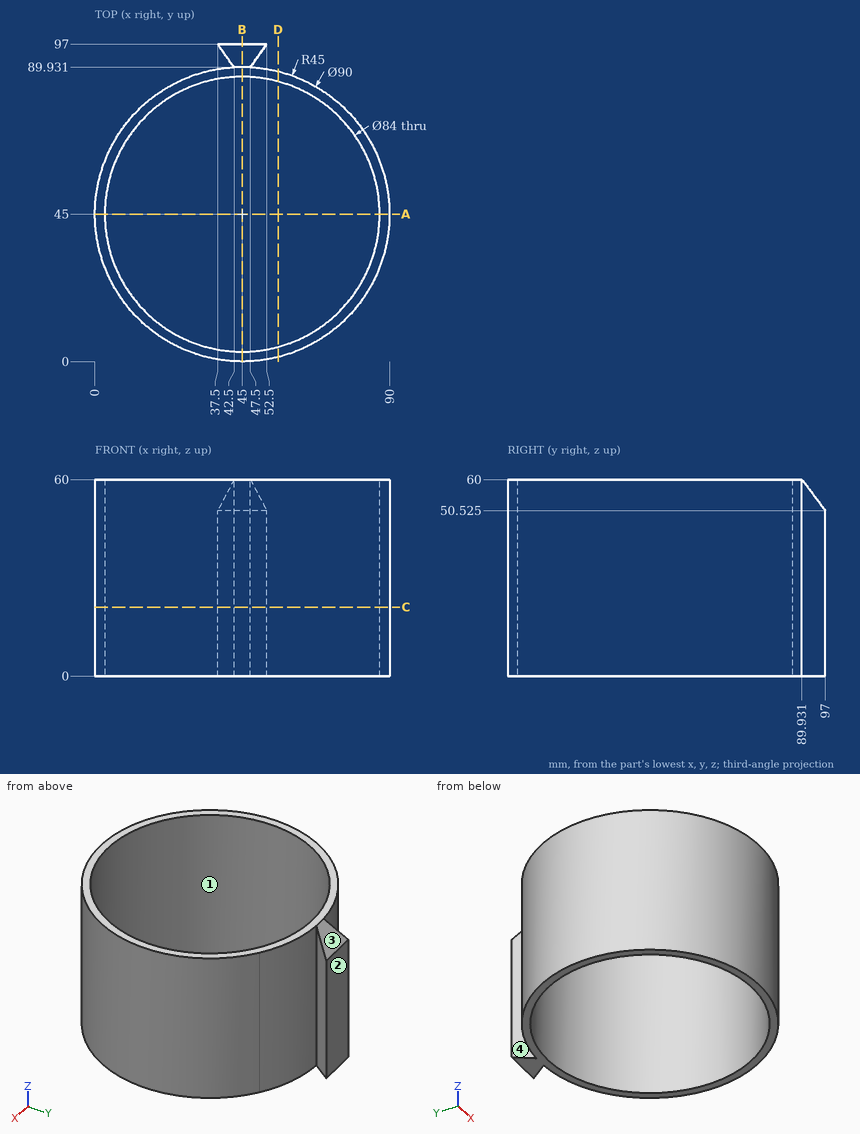
Verification items for this drawing (mm, ordinates from the low corner). A direction names the side the tool comes from. Coordinates: 2 decimals unless noted, no trailing zeros. Write each loop counter-clockwise with the first axis right and the second up, starting at its lowest first coordinate (ties: lowest second). Pieces come first, ordered by that corner, then holes. Notation, with made-up numbers: (-9, 13.5) -> (20, 13.5) arc R12 cw to (20, 17.5) -> close; hole circle Ø5 at (-37, -31). An arc over 180 degrees is marked (long way). One line per item, written item: value. Start each with the question number.
Q1. Cross-section at A-A on y = 45. Enter the section's corners in (x, z), and give its area (3 significant figures).
Q2. Cross-section at D-D on x = 56. Enter the section's corners in (y, z) (1 decimal).
Q3. Cross-section at B-B on x = 45. Enter the section's corners in (y, z) (1 decimal).
Q4. Cross-section at C-C on z = 21. Enter the section's corners in (x, y) (1 decimal).
Q5. Mould release check, pull along X, two halves, no side actions. Record for the marked faces 1 and 2: pulls with the +X half, pulls with the -X half, needs draft (parallel to the pull), parting line crosses it, or undercut.
Q6. Go/stop test with flat-tipped pins: P1, Ø5, axis at x = 72.5, z = 37, coming from the -Y side; P2, Ø3, axis at y = 27.5, z = 45, coming from the -X side; P3, Ø1.5, axis at x = 49, z = 28.5, coming from the -Y side. Record where each tip stops, or that it passes through.
Q7. Access from +Z, -Z, +X, -X, +Y, -Y to the whole of each face (thin tool, end or side, straight path). Record for the marked faces 3 and 4.
Q8. Thickness scan on L1, parallel to Y at x = 45, z = 25; L2, parallel to X at y = 73, z = 52 (1 decimal); L3, parallel to Y at x = 77.5, z = 54.5 (1 decimal). Record the ranges inside material, lowest first. Write a range as from..to.
Checked values:
1. outline: (0, 0) -> (3, 0) -> (3, 60) -> (0, 60) -> close; (87, 0) -> (90, 0) -> (90, 60) -> (87, 60) -> close
1. area: 360 mm²
2. outline: (1.4, 0) -> (4.5, 0) -> (4.5, 60) -> (1.4, 60) -> close; (85.5, 0) -> (88.6, 0) -> (88.6, 60) -> (85.5, 60) -> close
3. outline: (0, 0) -> (3, 0) -> (3, 60) -> (0, 60) -> close; (87, 0) -> (97, 0) -> (97, 50.5) -> (89.9, 60) -> (87, 60) -> close
4. outline: (37.5, 97) -> (42.5, 89.9) arc R45 ccw (long way) to (47.5, 89.9) -> (52.5, 97) -> close; hole circle Ø84 at (45, 45)
5. face 1: undercut
5. face 2: needs draft
6. P1: stops at y = 7.58
6. P2: stops at x = 2.94
6. P3: stops at y = 0.12
7. face 3: +Z, +X, -X, +Y
7. face 4: +Z, -Z, -X
8. L1: y = 0..3, 87..97
8. L2: x = 9.8..13.7, 76.3..80.2
8. L3: y = 13.9..18.4, 71.6..76.1
